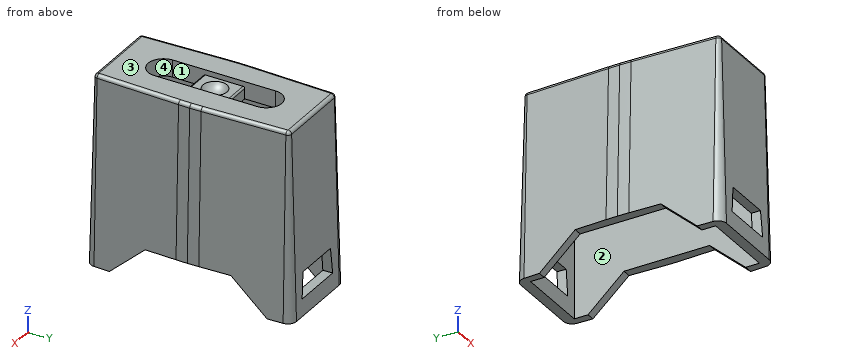
```python
from build123d import *

# Parameters (mm, degrees)
BOSS_EXTRUDE1_DEPTH = 13.97
BOSS_EXTRUDE1_TAPER = 1.5
SKETCH2_W           = 5.461
SKETCH2_H           = 13.716
CUT_EXTRUDE1_DEPTH  = 8.255
CUT_EXTRUDE2_DEPTH  = 18.403644698
SKETCH5_W           = 5.334
SKETCH5_H           = 3.048
BOSS_EXTRUDE2_DEPTH = 2.286
SKETCH7_W           = 1.778
SKETCH7_H           = 3.048
CUT_EXTRUDE5_DEPTH  = 4.445
SKETCH9_W           = 1.778
SKETCH9_H           = 2.54
SKETCH9_H_2         = 1.397
CUT_EXTRUDE6_DEPTH  = 1.524
FILLET2_RADIUS      = 0.889
FILLET2_LENGTH      = 1.397
FILLET3_RADIUS      = 0.889
FILLET3_LENGTH      = 2.54
FILLET4_RADIUS      = 0.889
FILLET4_LENGTH      = 1.397
FILLET5_R           = 0.254
FILLET6_R           = 0.127
CUT_EXTRUDE7_REACH  = 23.72
CUT_EXTRUDE8_REACH  = 23.712
CUT_EXTRUDE10_DEPTH = 18.403644779


with BuildPart() as part:
    # Sketch1 → Boss-Extrude1 (new body)
    with BuildSketch(Plane.XY):
        with BuildLine():
            ThreePointArc((6.827680219, 7.006153229), (6.634503314, 7.441430334), (6.193032647, 7.62))
            Line((6.193032647, 7.62), (0.868167353, 7.62))
            ThreePointArc((0.868167353, 7.62), (0.426696686, 7.441430334), (0.233519781, 7.006153229))
            Line((0.233519781, 7.006153229), (0.028202051, 0.84612915))
            ThreePointArc((0.028202051, 0.84612915), (0.017629462, 0.423123288), (0.01410494, 0))
            ThreePointArc((0.01410494, 0), (0.017629462, -0.423123288), (0.028202051, -0.84612915))
            Line((0.028202051, -0.84612915), (0.233519781, -7.006153229))
            ThreePointArc((0.233519781, -7.006153229), (0.426696686, -7.441430334), (0.868167353, -7.62))
            Line((0.868167353, -7.62), (6.193032647, -7.62))
            ThreePointArc((6.193032647, -7.62), (6.634503314, -7.441430334), (6.827680219, -7.006153229))
            Line((6.827680219, -7.006153229), (7.032997949, -0.84612915))
            ThreePointArc((7.032997949, -0.84612915), (7.043570538, -0.423123288), (7.04709506, 0))
            ThreePointArc((7.04709506, 0), (7.043570538, 0.423123288), (7.032997949, 0.84612915))
            Line((7.032997949, 0.84612915), (6.827680219, 7.006153229))
        make_face()
    extrude(amount=BOSS_EXTRUDE1_DEPTH, taper=BOSS_EXTRUDE1_TAPER)

    # Sketch2 → Cut-Extrude1 (cut)
    with BuildSketch(Plane(origin=(0, 0, 0), x_dir=(-1, 0, 0), z_dir=(0, 0, -1))):
        with Locations((-3.52354753, 0)):
            Rectangle(SKETCH2_W, SKETCH2_H)
    extrude(amount=-CUT_EXTRUDE1_DEPTH, mode=Mode.SUBTRACT)

    # Sketch3 → Cut-Extrude2 (cut, through all)
    with BuildSketch(Plane.XY.offset(13.97)):
        with BuildLine():
            Line((4.6736, 3.81), (4.6736, -3.81))
            ThreePointArc((4.6736, -3.81), (3.5306, -4.953), (2.3876, -3.81))
            Line((2.3876, -3.81), (2.3876, 3.81))
            ThreePointArc((2.3876, 3.81), (3.5306, 4.953), (4.6736, 3.81))
        make_face()
    extrude(amount=-CUT_EXTRUDE2_DEPTH, mode=Mode.SUBTRACT)

    # Sketch5 → Boss-Extrude2 (add)
    with BuildSketch(Plane.ZY.offset(-4.6736)):
        with Locations((10.922, 0)):
            Rectangle(SKETCH5_W, SKETCH5_H)
    extrude(amount=BOSS_EXTRUDE2_DEPTH)

    # Sketch6 → Cut-Revolve1 (revolve, cut)
    with BuildSketch(Plane(origin=(0, 0, 0), x_dir=(1, 0, 0), z_dir=(0, 1, 0)), mode=Mode.PRIVATE) as cut_revolve1_sk:
        with BuildLine():
            Line((3.5306, -13.589), (3.5306, -13.081))
            ThreePointArc((3.5306, -13.081), (3.018646633, -13.216956608), (2.6416, -13.589))
            Line((2.6416, -13.589), (3.5306, -13.589))
        make_face()
    revolve(cut_revolve1_sk.sketch.rotate(Axis((3.5306, 0, 13.589), (0, 0, -1)), 180), axis=Axis((3.5306, 0, 13.589), (0, 0, -1)), mode=Mode.SUBTRACT)

    # Sketch7 → Cut-Extrude5 (cut)
    with BuildSketch(Plane(origin=(0, 0, 8.255), x_dir=(-1, 0, 0), z_dir=(0, 0, -1))):
        Polygon((-1.06115247, -6.604), (-2.6416, -6.604), (-2.6416, -4.953), (-4.4196, -4.953), (-4.4196, -6.604), (-6.00004753, -6.604), (-6.00004753, 6.604), (-4.4196, 6.604), (-4.4196, 4.953), (-2.6416, 4.953), (-2.6416, 6.604), (-1.06115247, 6.604), align=None)
        with Locations((-3.5306, 0)):
            Rectangle(SKETCH7_W, SKETCH7_H, mode=Mode.SUBTRACT)
    extrude(amount=-CUT_EXTRUDE5_DEPTH, mode=Mode.SUBTRACT)

    # Sketch9 → Cut-Extrude6 (cut)
    with BuildSketch(Plane(origin=(0, 0, 8.255), x_dir=(-1, 0, 0), z_dir=(0, 0, -1))):
        with Locations((-3.5306, 0)):
            Rectangle(SKETCH9_W, SKETCH9_H)
        with Locations((-3.5306, 5.9055)):
            Rectangle(SKETCH9_W, SKETCH9_H_2)
        with Locations((-3.5306, -5.9055)):
            Rectangle(SKETCH9_W, SKETCH9_H_2)
    extrude(amount=-CUT_EXTRUDE6_DEPTH, mode=Mode.SUBTRACT)

    # Fillet2: full round fillet: the end face becomes a half cylinder, R = half its width
    fillet2_face = Plane((3.5306, -5.9055, 9.779), x_dir=(0, -1, 0), z_dir=(0, 0, -1))  # on the end face: x along it, z out of the body
    fillet2_slab = fillet2_face.offset(-FILLET2_RADIUS / 2) * Box(FILLET2_LENGTH, 2 * FILLET2_RADIUS, FILLET2_RADIUS, mode=Mode.PRIVATE)  # the body's end, R deep
    fillet2_round = Plane((3.5306, -5.9055, 10.668), x_dir=(0, 0, -1), z_dir=(0, -1, 0)) * Cylinder(FILLET2_RADIUS, FILLET2_LENGTH, mode=Mode.PRIVATE)  # its axis R under the face
    add(fillet2_slab - fillet2_round, mode=Mode.SUBTRACT)

    # Fillet3: full round fillet: the end face becomes a half cylinder, R = half its width
    fillet3_face = Plane((3.5306, 0, 9.779), x_dir=(0, -1, 0), z_dir=(0, 0, -1))  # on the end face: x along it, z out of the body
    fillet3_slab = fillet3_face.offset(-FILLET3_RADIUS / 2) * Box(FILLET3_LENGTH, 2 * FILLET3_RADIUS, FILLET3_RADIUS, mode=Mode.PRIVATE)  # the body's end, R deep
    fillet3_round = Plane((3.5306, 0, 10.668), x_dir=(0, 0, -1), z_dir=(0, -1, 0)) * Cylinder(FILLET3_RADIUS, FILLET3_LENGTH, mode=Mode.PRIVATE)  # its axis R under the face
    add(fillet3_slab - fillet3_round, mode=Mode.SUBTRACT)

    # Fillet4: full round fillet: the end face becomes a half cylinder, R = half its width
    fillet4_face = Plane((3.5306, 5.9055, 9.779), x_dir=(0, -1, 0), z_dir=(0, 0, -1))  # on the end face: x along it, z out of the body
    fillet4_slab = fillet4_face.offset(-FILLET4_RADIUS / 2) * Box(FILLET4_LENGTH, 2 * FILLET4_RADIUS, FILLET4_RADIUS, mode=Mode.PRIVATE)  # the body's end, R deep
    fillet4_round = Plane((3.5306, 5.9055, 10.668), x_dir=(0, 0, -1), z_dir=(0, -1, 0)) * Cylinder(FILLET4_RADIUS, FILLET4_LENGTH, mode=Mode.PRIVATE)  # its axis R under the face
    add(fillet4_slab - fillet4_round, mode=Mode.SUBTRACT)

    # Fillet5
    fillet5_edges = [part.edges().sort_by_distance(p)[0] for p in [
        (0.681023644, 7.178485258, 13.97),
        (0.49647521, 3.91395502, 13.97),
        (0.383396026, 0.417029358, 13.97),
        (0.49647521, -3.91395502, 13.97),
        (0.681023644, -7.178485258, 13.97),
        (3.5306, -7.254182676, 13.97),
        (6.380176356, -7.178485258, 13.97),
        (6.56472479, -3.91395502, 13.97),
        (6.677803974, -0.417029358, 13.97),
        (6.380176356, 7.178485258, 13.97),
        (6.56472479, 3.91395502, 13.97),
        (3.5306, 7.254182676, 13.97),
    ]]
    fillet(fillet5_edges, radius=FILLET5_R)

    # Fillet6
    fillet6_edges = [part.edges().sort_by_distance(p)[0] for p in [
        (3.5306, -1.524, 13.589),
        (3.5306, 1.524, 13.589),
    ]]
    fillet(fillet6_edges, radius=FILLET6_R)

    # Cut-Extrude7: up to this plane
    cut_extrude7_end = Plane(origin=(6.25404753, -6.858, 28.733169612), z_dir=(0, -1, 0))
    # Sketch10 → Cut-Extrude7 (cut, up to the surface)
    with BuildSketch(Plane(origin=(0, -7.614778527, 0.199399993), x_dir=(-1, 0, 0), z_dir=(0, -0.9996573249755574, 0.026176948307873222)), mode=Mode.PRIVATE) as cut_extrude7_sk1:
        Polygon((-1.6256, -1.070531654), (-5.4356, -1.070531654), (-5.2451, -2.975531654), (-1.8161, -2.975531654), align=None)
    cut_extrude7_tool1 = split(extrude(cut_extrude7_sk1.sketch, amount=CUT_EXTRUDE7_REACH, dir=(0, 1, 0), mode=Mode.PRIVATE), bisect_by=cut_extrude7_end, keep=Keep.BOTH, mode=Mode.PRIVATE)
    add(cut_extrude7_tool1.solids().sort_by_distance((3.5306, -7.562259, 2.205034))[0], mode=Mode.SUBTRACT)

    # Cut-Extrude8: up to this plane
    cut_extrude8_end = Plane(origin=(6.25404753, 6.858, 28.733169612), z_dir=(0, 1, 0))
    # Sketch12 → Cut-Extrude8 (cut, up to the surface)
    with BuildSketch(Plane(origin=(0, 7.614778527, 0.199399993), x_dir=(1, 0, 0), z_dir=(0, 0.9996573249755574, 0.026176948307873222)), mode=Mode.PRIVATE) as cut_extrude8_sk1:
        Polygon((5.4356, -1.070531654), (1.6256, -1.070531654), (1.8161, -2.975531654), (5.2451, -2.975531654), align=None)
    cut_extrude8_tool1 = split(extrude(cut_extrude8_sk1.sketch, amount=-CUT_EXTRUDE8_REACH, mode=Mode.PRIVATE), bisect_by=cut_extrude8_end, keep=Keep.BOTH, mode=Mode.PRIVATE)
    add(cut_extrude8_tool1.solids().sort_by_distance((3.5306, 7.562259, 2.205034))[0], mode=Mode.SUBTRACT)

    # Sketch13 → Cut-Extrude10 (cut, through all)
    with BuildSketch(Plane(origin=(0, 0, 0), x_dir=(0, 0, -1), z_dir=(1, 0, 0))):
        Polygon((0, 5.842), (0, -5.842), (-2.413, -3.175), (-2.413, 3.175), align=None)
    extrude(amount=CUT_EXTRUDE10_DEPTH, mode=Mode.SUBTRACT)


solid = part.part
```
Check sheet for the modelled part. Datum: model origin and axes. Units: mm. Face numbers are marked on the shaded views. A direction names the side the tool comes from. Give positions to 0.01 mm unless a question says otherwise; leave off trailing zeros. Order: outer loops, then holes, each group sorted by start corner. A loop starts at its lowest first (then second) coordinate and runs counter-clockwise, first axis right, second up. Notation, with made-up numbers: M 11.25,-32.75 L 66.25,-32.75 A23 cw 66.25,-5.75 Z; hole C 37.5,-3.75 d11. An arc over 180 degrees is marked long. Answer in a Markdown table with one row per item. Add a question column.
Q1. Access from +Z, -Z, +X, -X, +Y, -Y to the whole of each face (thin tool, end or side, straight path). Record for the marked faces 1 and 2.
Q2. Sectioned sample at C-C, the plane z = 4.5. Record the boundary of the cut face in (x, y) (3 decimals).
Q3. Sectioned sample at A-A, the plane z = 7. Record the boundary of the cut face in (x, y) (3 decimals), and give its area (3 significant figures).
Q4. Release check for a two-part mould opening along X. For the marked faces 3 and 4 record: released by +X, released by -X, zero draft, split by the parting line, or undercut.
Q5. Thickness scan on L1, parallel to X at y = 2, z = 4; L2, parallel to Y at x = 1.25, z = 3; L3, parallel to Z at x = 1.75, y = -1.5. Record the ranges inside material, lowest first.
Q6. Sectioned sample at B-B, the plane z = 12.25. Record the boundary of the cut face in (x, y) (3 decimals), and give its area (3 significant figures).
Q7. Gauge pin test, flat ends, axial feed: pin 1 Ø1 at (y, z) = (-2, 7) entering from -X; pin 2 Ø2.5 at (y, z) = (0, 10.5) entering from -X; pin 3 Ø1.5 at (x, z) = (1, 12) entering from -Y. Record the tip position at first contact, or that the pin passes through.
Verdict:
| question | item | result |
|---|---|---|
| 1 | face 1 | +Z |
| 1 | face 2 | -Z |
| 2 | outline | M 0.146,-0.842 L 0.351,-7.002 A0.517 ccw 0.868,-7.502 L 6.193,-7.502 A0.517 ccw 6.71,-7.002 L 6.915,-0.842 A25.282 ccw 6.915,0.842 L 6.71,7.002 A0.517 ccw 6.193,7.502 L 0.868,7.502 A0.517 ccw 0.351,7.002 L 0.146,0.842 A25.282 ccw Z; hole M 0.793,-6.858 L 6.254,-6.858 L 6.254,6.858 L 0.793,6.858 Z |
| 3 | outline | M 0.211,-0.84 L 0.417,-7 A0.452 ccw 0.868,-7.437 L 6.193,-7.437 A0.452 ccw 6.644,-7 L 6.85,-0.84 A25.217 ccw 6.85,0.84 L 6.644,7 A0.452 ccw 6.193,7.437 L 0.868,7.437 A0.452 ccw 0.417,7 L 0.211,0.84 A25.217 ccw Z; hole M 0.793,-6.858 L 6.254,-6.858 L 6.254,6.858 L 0.793,6.858 Z |
| 3 | area | 20.8 mm² |
| 4 | face 3 | zero draft |
| 4 | face 4 | undercut |
| 5 | L1 | 0.17 to 0.79, 6.25 to 6.89 |
| 5 | L2 | -7.54 to -6.86, 6.86 to 7.54 |
| 5 | L3 | 12.7 to 13.97 |
| 6 | outline | M 0.349,-0.835 L 0.554,-6.995 A0.314 ccw 0.868,-7.299 L 6.193,-7.299 A0.314 ccw 6.507,-6.995 L 6.712,-0.835 A25.079 ccw 6.712,0.835 L 6.507,6.995 A0.314 ccw 6.193,7.299 L 0.868,7.299 A0.314 ccw 0.554,6.995 L 0.349,0.835 A25.079 ccw Z; M 2.642,-1.524 L 4.42,-1.524 L 4.42,1.524 L 2.642,1.524 Z; hole M 1.061,-6.604 L 2.642,-6.604 L 2.642,-4.953 L 4.42,-4.953 L 4.42,-6.604 L 6,-6.604 L 6,6.604 L 4.42,6.604 L 4.42,4.953 L 2.642,4.953 L 2.642,6.604 L 1.061,6.604 Z |
| 6 | area | 36.1 mm² |
| 7 | pin 1 | x = 0.23 |
| 7 | pin 2 | x = 0.26 |
| 7 | pin 3 | y = -7.33 |
